from build123d import *

# Parameters (mm, degrees)
BOSS_EXTRUDE2_DEPTH      = 3.4
BOSS_EXTRUDE2_DEPTH_BACK = 3.4
SKETCH1_W                = 29.999999097
SKETCH1_H                = 9.300000034
SKETCH3_W                = 7.5
SKETCH3_H                = 3.300000034
CUT_EXTRUDE1_DEPTH       = 6.8
SKETCH4_W                = 7.5
SKETCH4_H                = 3.300000034
CUT_EXTRUDE2_DEPTH       = 6.8
BOSS_EXTRUDE3_START      = -3
BOSS_EXTRUDE3_DEPTH      = 3
BOSS_EXTRUDE4_START      = -3
BOSS_EXTRUDE4_DEPTH      = 3
BOSS_EXTRUDE5_START      = -3
BOSS_EXTRUDE5_DEPTH      = 3
BOSS_EXTRUDE6_START      = -3
BOSS_EXTRUDE6_DEPTH      = 3
CUT_EXTRUDE3_START       = -9.3
SKETCH9_R                = 1.39
CUT_EXTRUDE3_DEPTH       = 9.3
CUT_EXTRUDE4_START       = -9.3
SKETCH10_R               = 1.39
CUT_EXTRUDE4_DEPTH       = 9.3


with BuildPart() as part:
    # Sketch1 → Boss-Extrude2 (new, two sides: drawn at the far end of the back side and taken through both)
    with BuildSketch(Plane.XY.offset(-BOSS_EXTRUDE2_DEPTH_BACK)):
        with Locations((18.399999593, -4.650000017)):
            Rectangle(SKETCH1_W, SKETCH1_H)
    extrude(amount=BOSS_EXTRUDE2_DEPTH + BOSS_EXTRUDE2_DEPTH_BACK)

    # Sketch3 → Cut-Extrude1 (cut)
    with BuildSketch(Plane.XY.offset(3.4)):
        with Locations((7.150000045, -4.650000017)):
            Rectangle(SKETCH3_W, SKETCH3_H)
    extrude(amount=-CUT_EXTRUDE1_DEPTH, mode=Mode.SUBTRACT)

    # Sketch4 → Cut-Extrude2 (cut)
    with BuildSketch(Plane.XY.offset(3.4)):
        with Locations((29.649999142, -4.650000017)):
            Rectangle(SKETCH4_W, SKETCH4_H)
    extrude(amount=-CUT_EXTRUDE2_DEPTH, mode=Mode.SUBTRACT)

    # Sketch5 → Boss-Extrude3 (add)
    with BuildSketch(Plane(origin=(0, 0, 0), x_dir=(1, 0, 0), z_dir=(0, 1, 0)).offset(BOSS_EXTRUDE3_START)):
        with BuildLine():
            Line((3.400000045, 3.4), (3.400000045, -3.4))
            ThreePointArc((3.400000045, -3.4), (4.5e-08, 0), (3.400000045, 3.4))
        make_face()
    extrude(amount=BOSS_EXTRUDE3_DEPTH)

    # Sketch6 → Boss-Extrude4 (add)
    with BuildSketch(Plane(origin=(0, 0, 0), x_dir=(1, 0, 0), z_dir=(0, 1, 0)).offset(BOSS_EXTRUDE4_START)):
        with BuildLine():
            Line((33.399999142, 3.4), (33.399999142, -3.4))
            ThreePointArc((33.399999142, -3.4), (36.799999142, 0), (33.399999142, 3.4))
        make_face()
    extrude(amount=BOSS_EXTRUDE4_DEPTH)

    # Sketch7 → Boss-Extrude5 (add)
    with BuildSketch(Plane(origin=(0, -9.300000034, 0), x_dir=(-1, 0, 0), z_dir=(0, -1, 0)).offset(BOSS_EXTRUDE5_START)):
        with BuildLine():
            Line((-3.400000045, -3.4), (-3.400000045, 3.4))
            ThreePointArc((-3.400000045, 3.4), (-4.5e-08, 0), (-3.400000045, -3.4))
        make_face()
    extrude(amount=BOSS_EXTRUDE5_DEPTH)

    # Sketch8 → Boss-Extrude6 (add)
    with BuildSketch(Plane(origin=(0, -9.300000034, 0), x_dir=(-1, 0, 0), z_dir=(0, -1, 0)).offset(BOSS_EXTRUDE6_START)):
        with BuildLine():
            Line((-33.399999142, -3.4), (-33.399999142, 3.4))
            ThreePointArc((-33.399999142, 3.4), (-36.799999142, 0), (-33.399999142, -3.4))
        make_face()
    extrude(amount=BOSS_EXTRUDE6_DEPTH)

    # Sketch9 → Cut-Extrude3 (cut)
    with BuildSketch(Plane(origin=(0, 0, 0), x_dir=(1, 0, 0), z_dir=(0, 1, 0)).offset(CUT_EXTRUDE3_START)):
        with Locations(Location((3.400000045, 0, 0), (0, 0, 270))):
            Circle(SKETCH9_R)
    extrude(amount=CUT_EXTRUDE3_DEPTH, mode=Mode.SUBTRACT)

    # Sketch10 → Cut-Extrude4 (cut)
    with BuildSketch(Plane(origin=(0, 0, 0), x_dir=(1, 0, 0), z_dir=(0, 1, 0)).offset(CUT_EXTRUDE4_START)):
        with Locations(Location((33.399999142, 0, 0), (0, 0, 270))):
            Circle(SKETCH10_R)
    extrude(amount=CUT_EXTRUDE4_DEPTH, mode=Mode.SUBTRACT)


solid = part.part
Read the model definition and answer for the solid it produces. Units are mm, in the model's axes. A direction names the side the tool comes from. Round coordinates to 2 decimals unless told otherwise and drop trailing zeros. Order: outer loops, then holes, each group sorted by start corner. A loop starts at its lowest first (then second) coordinate and runs counter-clockwise, first axis right, second up.
1) The part is cut by section B-B on x = 31. Write down the section's boundary in (y, z).
2) Flat-ended cylindrical pins translate along their axes: pin 1 (1.7 mm diameter, centred on y = -5, z = -1, fed in from +X); pin 2 (1 mm diameter, centred on x = 4, y = -5, fed in from +Z). Find the tip coordinate at first contact, or state that the pin passes through.
3) The part is cut by section D-D on z = -3. Write down the section's boundary in (x, y).
4) The mould has two halves that part along X. Classify faces 4 (the face through (5, -6.3, 0)), 5 (the face through (2.043, -1.521, -0.301)), 6 (the face through (25.9, -5, 0)): released by +X, released by -X, zero draft, split by the parting line, or undercut.
5) The part is cut by section C-C on y = -8.5. Write down the section's boundary in (x, z).
6) The part is cut by section A-A on z = 0. Write down the section's boundary in (x, y), plus the area to 3 significant figures.
7) Straight lines are drawn through the part: L1, parallel to X at y = -1.5, z = 0; L2, parallel to Z at x = 33.4, y = -7.2; L3, parallel to Y at x = 28, z = -0.5. For each, find the intervals that lie inside material, in ascending order.
8) For faces 1 (the face through (31, -6.3, 0)), 2 (the face through (36.8, -7.8, -0.1)), 3 (the face through (6, -3, 0)), determine the directions among +Z, -Z, +X, -X, +Y, -Y from which every point of the face is accessible in a straight line to the end or side of a thin tool.
Resolved:
1. outline: (-9.3, -3.4) - (-6.3, -3.4) - (-6.3, 3.4) - (-9.3, 3.4) - close; (-3, -3.4) - (0, -3.4) - (0, 3.4) - (-3, 3.4) - close
2. pin 1: stops at x = 25.9
2. pin 2: passes through
3. outline: (1.8, -9.3) - (35, -9.3) - (35, -6.3) - (25.9, -6.3) - (25.9, -3) - (35, -3) - (35, 0) - (1.8, 0) - (1.8, -3) - (10.9, -3) - (10.9, -6.3) - (1.8, -6.3) - close
4. face 4: zero draft
4. face 5: undercut
4. face 6: released by +X
5. outline: (3.4, -3.4) - (33.4, -3.4) arc R3.4 ccw to (33.4, 3.4) - (3.4, 3.4) arc R3.4 ccw to start; hole circle Ø2.78 at (3.4, 0); hole circle Ø2.78 at (33.4, 0)
6. outline: (0, -9.3) - (2.01, -9.3) - (2.01, -6.3) - (0, -6.3) - close; (0, -3) - (2.01, -3) - (2.01, 0) - (0, 0) - close; (4.79, -9.3) - (32.01, -9.3) - (32.01, -6.3) - (25.9, -6.3) - (25.9, -3) - (32.01, -3) - (32.01, 0) - (4.79, 0) - (4.79, -3) - (10.9, -3) - (10.9, -6.3) - (4.79, -6.3) - close; (34.79, -9.3) - (36.8, -9.3) - (36.8, -6.3) - (34.79, -6.3) - close; (34.79, -3) - (36.8, -3) - (36.8, 0) - (34.79, 0) - close
6. area: 237 mm2
7. L1: x = 0 to 2.01, 4.79 to 32.01, 34.79 to 36.8
7. L2: z = -3.4 to -1.39, 1.39 to 3.4
7. L3: y = -9.3 to -6.3, -3 to 0
8. face 1: +Z, -Z, +X
8. face 2: +X, +Y, -Y
8. face 3: +Z, -Z, -X
